from build123d import *

# Parameters (mm, degrees)
F1_DEPTH     = 32
F3_DEPTH     = 64
F4_W         = 3.5
F4_H         = 35
F5_DEPTH     = 10.5
F7_DEPTH     = 3.5
F8_W         = 16
F8_H         = 4
F9_DEPTH     = 10.5
F10_T1_DEPTH = 48
F10_T3_DEPTH = 94
F11_W        = 35
F11_H        = 25
F12_DEPTH    = 4.001
F13_R        = 2


# Not quite as in the source:
# - a fillet or chamfer that OpenCascade refuses, or shapes differently, is made with other operations: its cross-section is extruded or revolved along the edge and cut away or added
# - a pattern or mirror of a feature is missing from the dataset's text; its kind, count and spacing are read off the source's solid


with BuildPart() as f1:
    # F0 (on Right) → F1 (new body, symmetric)
    with BuildSketch(Plane.YZ):
        Polygon((13.5, -6), (-22.5, -6), (-23.5, -5), (-23.5, -9), (17.5, -9), (17.5, 9), (-17.5, 9), (-17.5, 6), (-16.5, 7), align=None)
    extrude(amount=F1_DEPTH, both=True)

    # F2 (on face) → F3 (cut, through all)
    with BuildSketch(Plane.YZ.offset(32)):
        with BuildLine():
            Line((3.5, -1.6666666667), (13.5, -6))
            Line((13.5, -6), (13.5, -3.6666666667))
            ThreePointArc((13.5, -3.6666666667), (12.9142135624, -2.2524531043), (11.5, -1.6666666667))
            Line((11.5, -1.6666666667), (3.5, -1.6666666667))
        make_face()
    extrude(amount=-F3_DEPTH, mode=Mode.SUBTRACT)

    # F4 (on face) → F5 (join)
    with BuildSketch(Plane.XY.offset(9)):
        with Locations((-9.75, 0)):
            Rectangle(F4_W, F4_H)
    f5 = extrude(amount=F5_DEPTH)

    # F5_copies: F5 across plane
    add(f5.mirror(Plane(origin=(0, 0, 0), x_dir=(0, 0, 1), z_dir=(1, 0, 0))))

    # F6 (on face) → F7 (cut, through all)
    with BuildSketch(Plane(origin=(-11.5, 0, 0), x_dir=(0, -1, 0), z_dir=(-1, 0, 0))):
        with BuildLine():
            Line((13, 15.85), (-13, 15.85))
            ThreePointArc((-13, 15.85), (-13.7071067812, 15.5571067812), (-14, 14.85))
            Line((-14, 14.85), (-14, 13.65))
            ThreePointArc((-14, 13.65), (-13.7071067812, 12.9428932188), (-13, 12.65))
            Line((-13, 12.65), (13, 12.65))
            ThreePointArc((13, 12.65), (13.7071067812, 12.9428932188), (14, 13.65))
            Line((14, 13.65), (14, 14.85))
            ThreePointArc((14, 14.85), (13.7071067812, 15.5571067812), (13, 15.85))
        make_face()
    f7 = extrude(amount=-F7_DEPTH, mode=Mode.SUBTRACT)

    # F7_copies: F7 across plane
    add(f7.mirror(Plane(origin=(0, 0, 0), x_dir=(0, 0, 1), z_dir=(1, 0, 0))), mode=Mode.SUBTRACT)

    # F8 (on face) → F9 (join, through all)
    with BuildSketch(Plane.XY.offset(9)):
        with Locations((0, -15.5)):
            Rectangle(F8_W, F8_H)
    extrude(amount=F9_DEPTH)

    # F10: fillet of radius 6 on 3 edges, made by hand

    # F10_s2 → F10_t1 (cut)
    with BuildSketch(Plane.XY.offset(-24)):
        with BuildLine():
            ThreePointArc((26, 17.5), (30.2426406871, 15.7426406871), (32, 11.5))
            Line((32, 11.5), (32, 17.5))
            Line((32, 17.5), (26, 17.5))
        make_face()
        with BuildLine():
            ThreePointArc((-26, 17.5), (-30.2426406871, 15.7426406871), (-32, 11.5))
            Line((-32, 11.5), (-32, 17.5))
            Line((-32, 17.5), (-26, 17.5))
        make_face()
    extrude(amount=F10_T1_DEPTH, mode=Mode.SUBTRACT)

    # F10_s4 → F10_t3 (cut)
    with BuildSketch(Plane.YZ.offset(-47)):
        with BuildLine():
            ThreePointArc((17.5, -3), (15.7426406871, -7.2426406871), (11.5, -9))
            Line((11.5, -9), (17.5, -9))
            Line((17.5, -9), (17.5, -3))
        make_face()
    extrude(amount=F10_T3_DEPTH, mode=Mode.SUBTRACT)

    # F11 (on face) → F12 (cut, through all)
    with BuildSketch(Plane(origin=(0, 0, -9), x_dir=(1, 0, 0), z_dir=(0, 0, -1))):
        with Locations((0, 11)):
            Rectangle(F11_W, F11_H)
    extrude(amount=-F12_DEPTH, mode=Mode.SUBTRACT)

    # F13
    f13_edges = [f1.edges().sort_by_distance(p)[0] for p in [
        (0, 13.5, -6),
    ]]
    fillet(f13_edges, radius=F13_R)


solid = f1.part
Geometry check sheet. Reference: the model listing, model coordinates, mm. A direction names the side the tool comes from. Round coordinates to 2 decimals unless told otherwise and drop trailing zeros. Order: outer loops, then holes, each group sorted by start corner. A loop starts at its lowest first (then second) coordinate and runs counter-clockwise, first axis right, second up. Notation, with made-up numbers: (41, -25.5) -> (84, -25.5) arc R23 ccw to (84, -0.5) -> close; hole circle Ø7 at (-27, 58.25). An arc over 180 degrees is marked (long way). Use one line per item in the form item = value.
1. Scan lines: line 1 along X through (y, z) = (10.5, 18); line 2 along Z through (x, y) = (17, 11); line 3 along Z through (x, y) = (-20, -18.5). Record each from-to range of solid material in increasing order. Write a range as from..to.
Working result:
line_1 = -11.5..-8, 8..11.5
line_2 = -9..-6, -1.67..9
line_3 = -9..-6
2. Cross-section at C-C, the plane x = -13. Enter the section's corners in (y, z), plus the area to 3 significant figures.
Working result:
outline = (-17.5, 6) -> (-16.5, 7) -> (3.5, -1.67) -> (11.5, -1.67) arc R2 cw to (13.5, -3.67) -> (13.5, -4) arc R2 cw to (11.5, -6) -> (1.5, -6) -> (1.5, -9) -> (11.5, -9) arc R6 ccw to (17.5, -3) -> (17.5, 9) -> (-17.5, 9) -> close
area = 338 mm^2
3. Cross-section at B-B, the plane z = 12. Enter the section's corners in (x, y), plus the area to 3 significant figures.
Working result:
outline = (-11.5, -17.5) -> (11.5, -17.5) -> (11.5, 17.5) -> (8, 17.5) -> (8, -13.5) -> (-8, -13.5) -> (-8, 17.5) -> (-11.5, 17.5) -> close
area = 309 mm^2
4. Set-up check for faces 5 (the face through (11.5, 0, 12)), 6 (the face through (10, 0, 12.65)), 7 (the face through (0, -17.5, 11)), 8 (the face through (-8, 2, 12)): record each of +Z, -Z, +X, -X, +Y, -Y from which the full face is reachable in a straight line by a thin tool's end or side.
Working result:
face_5 = +Z, +X, +Y, -Y
face_6 = +X, -X
face_7 = +Z, +X, -X, -Y
face_8 = +Z, +Y
5. Mould release check, pull along Z, two halves, no side actions. Record for faces 1 (the face through (-9, -4, 19.5)), 2 (the face through (0, 1.5, -8)), 3 (the face through (0, 8, -1.667)), 4 (the face through (0, 2, -9)): pulls with the +Z half, pulls with the -Z half, needs draft (parallel to the pull), parting line crosses it, or undercut.
Working result:
face_1 = pulls with the +Z half
face_2 = needs draft
face_3 = undercut
face_4 = pulls with the -Z half
6. Cross-section at A-A, the plane y = 4.5. Enter the section's corners in (x, z), plus the area to 3 significant figures.
Working result:
outline = (-32, -9) -> (32, -9) -> (32, -6) -> (-32, -6) -> close; (-32, -1.67) -> (32, -1.67) -> (32, 9) -> (11.5, 9) -> (11.5, 12.65) -> (8, 12.65) -> (8, 9) -> (-8, 9) -> (-8, 12.65) -> (-11.5, 12.65) -> (-11.5, 9) -> (-32, 9) -> close; (-11.5, 15.85) -> (-8, 15.85) -> (-8, 19.5) -> (-11.5, 19.5) -> close; (8, 15.85) -> (11.5, 15.85) -> (11.5, 19.5) -> (8, 19.5) -> close
area = 926 mm^2
7. Go/stop test with flat-tipped pins: pin 1 (5 mm diameter, centred on x = -17, y = -7.5, fed in from +Z); pin 2 (3.5 mm diameter, centred on x = 4.5, z = -7, fed in from -Y); pin 3 (8.5 mm diameter, centred on y = 6.5, z = 16.5, fed in from -X). Record where each tip stops, or that it passes through.
Working result:
pin_1 = 9
pin_2 = 1.5
pin_3 = -11.5
8. Cross-section at D-D, the plane y = -5. Enter the section's corners in (x, z), plus the area to 3 significant figures.
Working result:
outline = (-32, -9) -> (-17.5, -9) -> (-17.5, -6) -> (-32, -6) -> close; (-32, 2.02) -> (32, 2.02) -> (32, 9) -> (11.5, 9) -> (11.5, 12.65) -> (8, 12.65) -> (8, 9) -> (-8, 9) -> (-8, 12.65) -> (-11.5, 12.65) -> (-11.5, 9) -> (-32, 9) -> close; (-11.5, 15.85) -> (-8, 15.85) -> (-8, 19.5) -> (-11.5, 19.5) -> close; (8, 15.85) -> (11.5, 15.85) -> (11.5, 19.5) -> (8, 19.5) -> close; (17.5, -9) -> (32, -9) -> (32, -6) -> (17.5, -6) -> close
area = 585 mm^2
